The listing builds one solid part. Answer for the finished solid, in the listing's coordinates (mm). A direction names the side the tool comes from. Coordinates: 2 decimals unless noted, no trailing zeros. Order: outer loops, then holes, each group sorted by start corner. A loop starts at its lowest first (then second) coordinate and runs counter-clockwise, first axis right, second up. Notation, with made-up numbers: (2.5, 85) -> (29.5, 85) arc R10 cw to (29.5, 90) -> close; hole circle Ø1 at (30, 30.5). An arc over 180 degrees is marked (long way). Return JSON: item names as keys, results as strings.
```python
from build123d import *

# Parameters (mm, degrees)
SHELL2_T           = -10
SKETCH6_W          = 12
SKETCH6_H          = 25
CUT_EXTRUDE2_DEPTH = 47.434654221
SKETCH7_R          = 1
CUT_EXTRUDE3_DEPTH = 5


with BuildPart() as part:
    # Sketch5 → Revolve3 (revolve)
    with BuildSketch(Plane.XY, mode=Mode.PRIVATE) as revolve3_sk:
        Polygon((0, 0), (0, 18.872655155), (-18, 18.872655155), (-30, 0), align=None)
    revolve(revolve3_sk.sketch.rotate(Axis((0, 0, 0), (0, 1, 0)), 270), axis=Axis((0, 0, 0), (0, 1, 0)))

    # Shell2
    shell2_openings = [part.faces().sort_by_distance(p)[0] for p in [
        (0, 0, 0),
    ]]
    offset(amount=SHELL2_T, openings=shell2_openings, kind=Kind.INTERSECTION)

    # Sketch6 → Cut-Extrude2 (cut, through all)
    with BuildSketch(Plane(origin=(0, 18.872655155, 0), x_dir=(1, 0, 0), z_dir=(0, 1, 0))):
        Rectangle(SKETCH6_W, SKETCH6_H)
    extrude(amount=-CUT_EXTRUDE2_DEPTH, mode=Mode.SUBTRACT)

    # Sketch7 → Cut-Extrude3 (cut)
    with BuildSketch(Plane(origin=(0, 18.872655155, 0), x_dir=(1, 0, 0), z_dir=(0, 1, 0))):
        with Locations(Location((0, 13.7, 0), (0, 0, 270))):
            Circle(SKETCH7_R)
        with Locations(Location((0, -14.3, 0), (0, 0, 270))):
            Circle(SKETCH7_R)
    extrude(amount=-CUT_EXTRUDE3_DEPTH, mode=Mode.SUBTRACT)


solid = part.part
```
Item 1: The part is cut by section B-B on y = 15.75. Determine the outline of the cut face in (x, z), plus the area to 3 significant figures.
Answer list:
{"outline": "circle Ø39.97 at (0, 0); hole (-6, -12.5) -> (6, -12.5) -> (6, 12.5) -> (-6, 12.5) -> close; hole circle Ø2 at (0, -13.7); hole circle Ø2 at (0, 14.3)", "area": "949 mm2"}
Item 2: The part is cut by section A-A on z = 0. Determine the outline of the cut face in (x, y), plus the area to 3 significant figures.
Answer list:
{"outline": "(-30, 0) -> (-18.15, 0) -> (-12.51, 8.87) -> (-6, 8.87) -> (-6, 18.87) -> (-18, 18.87) -> close; (6, 8.87) -> (12.51, 8.87) -> (18.15, 0) -> (30, 0) -> (18, 18.87) -> (6, 18.87) -> close", "area": "514 mm2"}
Item 3: Determine the mould class of faces 1 (the conical face through (18.305, 17.692, 4.065)), 2 (the cylindrical face through (-0.383, 16.408, 15.224)), 3 (the conical face through (-0.565, 8.318, 12.849)), 4 (the flat face through (8, 18.873, 0)) for opening direction X: pulls with the +X half, pulls with the -X half, needs draft (parallel to the pull), parting line crosses it, or undercut.
Answer list:
{"face 1": "parting line crosses it", "face 2": "undercut", "face 3": "undercut", "face 4": "needs draft"}
Item 4: Flat-ended cylindrical pins translate along their axes: pin 1 (1 mm diameter, centred on x = -1, y = 13, fed in from +Z); pin 2 (6 mm diameter, centred on x = -3, y = 16, fed in from +Z); pin 3 (2 mm diameter, centred on x = 8, y = 16.5, fed in from +Z). Find the tip coordinate at first contact, or state that the pin passes through.
Answer list:
{"pin 1": "z = 22.03", "pin 2": "z = 21.56", "pin 3": "z = 18.6"}
Item 5: The part is cut by section C-C on y = 2.5. Determine the outline of the cut face in (x, z), plus the area to 3 significant figures.
Answer list:
{"outline": "circle Ø56.82 at (0, 0); hole circle Ø33.12 at (0, 0)", "area": "1,670 mm2"}
Item 6: Find the intervals of material crossed by probe 1 along X at (y, z) = (6.25, 10.5); probe 2 along X at (y, z) = (16.6, 14.3); probe 3 along X at (y, z) = (9, -15), in increasing order.
Answer list:
{"probe 1": "-23.81 to -9.52, 9.52 to 23.81", "probe 2": "-13.18 to -1, 1 to 13.18", "probe 3": "-19.09 to 19.09"}
Item 7: Which of the six approach directions +Z, -Z, +X, -X, +Y, -Y give full straight-line access (tool end or side, diameter ignored) to faces 5 (the flat face through (-9, 8.873, 0)), 6 (the flat face through (6, 14, 0)), 7 (the flat face through (0, 13.873, -14))?
Answer list:
{"face 5": "-Y", "face 6": "+Y, -Y", "face 7": "+Y"}
